Could you check a few things on this model? Use its own coordinates, in mm. Round coordinates to 2 decimals unless told otherwise and drop trailing zeros. Loops run counter-clockwise (first coordinate to the right, second up) from the corner with the lowest first, then second, coordinate; pieces in that order, holes last. Notation, with made-up numbers: (19.5, -28) -> (44.5, -28) arc R12 cw to (44.5, -20) -> close; hole circle Ø6 at (-34, 57.5). An arc over 180 degrees is marked (long way). One line per item, written item: value.
from build123d import *

# Parameters (mm, degrees)
F0_W     = 29
F0_H     = 29
F1_DEPTH = 1.5
F2_R     = 8.5
F3_DEPTH = 1.501
F4_R     = 1
F5_DEPTH = 1.501
F6_W     = 1.5
F6_H     = 1.5
F6_H_2   = 10
F7_DEPTH = 1.5


# Not quite as in the source:
# - a pattern or mirror of a feature is missing from the dataset's text; its kind, count and spacing are read off the source's solid


with BuildPart() as f1:
    # F0 (on Front) → F1 (new body)
    with BuildSketch(Plane.XZ):
        Rectangle(F0_W, F0_H)
    extrude(amount=F1_DEPTH)

    # F2 (on face) → F3 (cut, through all)
    with BuildSketch(Plane.XZ.offset(1.5)):
        Circle(F2_R)
    extrude(amount=-F3_DEPTH, mode=Mode.SUBTRACT)

    # F4 (on face) → F5 (cut, through all)
    with BuildSketch(Plane.XZ.offset(1.5)):
        with Locations((-10, 0)):
            Circle(F4_R)
    f5 = extrude(amount=-F5_DEPTH, mode=Mode.SUBTRACT)

    # F5_copies: F5 across plane
    add(f5.mirror(Plane(origin=(0, 0, 0), x_dir=(0, 0, 1), z_dir=(1, 0, 0))), mode=Mode.SUBTRACT)

    # F6 (on face) → F7 (join)
    with BuildSketch(Plane.XZ.offset(1.5)):
        with Locations((-15.25, -13)):
            Rectangle(F6_W, F6_H)
        with Locations((-15.25, 7)):
            Rectangle(F6_W, F6_H_2)
    f7 = extrude(amount=-F7_DEPTH)

    # F7_copies: F7 across plane
    add(f7.mirror(Plane(origin=(0, 0, 0), x_dir=(0, 0, 1), z_dir=(1, 0, 0))))


solid = f1.part
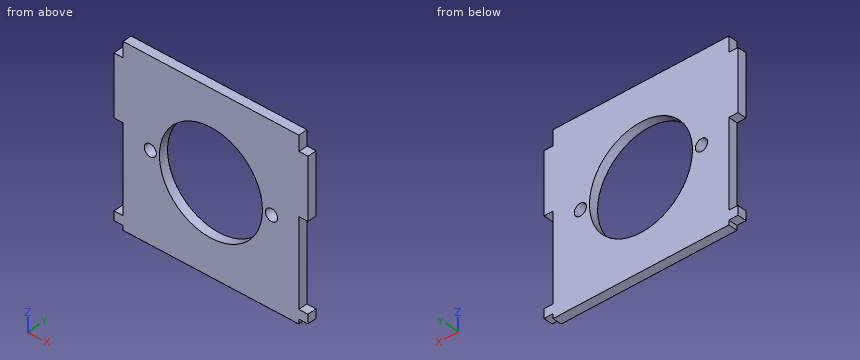
(1) If I drill on L1, parallel to Z at x = 10, y = -0.75; L2, parallel to Z at x = 0, y = -1.05; L3, parallel to X at y = -0.6, z = 13.75, over which ranges is the centre line in solid material (lowest first)?
Recorded:
L1: -14.5 to -1, 1 to 14.5
L2: -14.5 to -8.5, 8.5 to 14.5
L3: -14.5 to 14.5
(2) If we section it at C-C, the plane z = 0: Please give me the cut outline in (x, y).
Recorded:
outline: (-14.5, -1.5) -> (-11, -1.5) -> (-11, 0) -> (-14.5, 0) -> close; (-9, -1.5) -> (-8.5, -1.5) -> (-8.5, 0) -> (-9, 0) -> close; (8.5, -1.5) -> (9, -1.5) -> (9, 0) -> (8.5, 0) -> close; (11, -1.5) -> (14.5, -1.5) -> (14.5, 0) -> (11, 0) -> close
(3) I'm going to push flat-ended pins straight in: pin 1 Ø0.8 at (x, y) = (-15, -0.5) entering from -Z; pin 2 Ø0.8 at (x, y) = (-15, -0.5) entering from +Z; pin 3 Ø1.8 at (x, z) = (10, 0) entering from +Y; pin 4 Ø0.8 at (y, z) = (-0.5, 13.5) entering from +X. Where does each tip first touch, or does it pass through?
Recorded:
pin 1: z = -13.75
pin 2: z = 12
pin 3: through
pin 4: x = 14.5
(4) If we section it at D-D, the plane y = -0.6: Please give me the cut outline in (x, z), then the cut area to 3 significant figures.
Recorded:
outline: (-16, -13.75) -> (-14.5, -13.75) -> (-14.5, -14.5) -> (14.5, -14.5) -> (14.5, -13.75) -> (16, -13.75) -> (16, -12.25) -> (14.5, -12.25) -> (14.5, 2) -> (16, 2) -> (16, 12) -> (14.5, 12) -> (14.5, 14.5) -> (-14.5, 14.5) -> (-14.5, 12) -> (-16, 12) -> (-16, 2) -> (-14.5, 2) -> (-14.5, -12.25) -> (-16, -12.25) -> close; hole circle Ø2 at (-10, 0); hole circle Ø17 at (0, 0); hole circle Ø2 at (10, 0)
area: 642 mm²
(5) If we section it at B-B, the plane z = 7.5: Please give me the cut outline in (x, y), then the cut area to 3 significant figures.
Recorded:
outline: (-16, -1.5) -> (-4, -1.5) -> (-4, 0) -> (-16, 0) -> close; (4, -1.5) -> (16, -1.5) -> (16, 0) -> (4, 0) -> close
area: 36.0 mm²
(6) If we section it at A-A, the plane x = 4: Please give me the cut outline in (y, z).
Recorded:
outline: (-1.5, -14.5) -> (0, -14.5) -> (0, -7.5) -> (-1.5, -7.5) -> close; (-1.5, 7.5) -> (0, 7.5) -> (0, 14.5) -> (-1.5, 14.5) -> close
